Answer from the drawing. Dimensions are ordinates in mm from the lowest x, y and z of the part. Round coordinates to 2 decimals unless told otherwise and drop trailing zeros. Order: outer loops, then holes, each group sorted by start corner. A loop starts at its lowest first (then second) coordinate and runs counter-clockwise, first axis right, second up. Notation, with made-up numbers: (4.25, 43.25) -> (13.25, 43.25) arc R18 ccw to (13.25, 54.25) -> close; hole circle Ø4 at (57, 80). An arc over 180 degrees is marked (long way). Use a Markdown table: item, result. Add a question column.
1. Section D-D, the plane x = 2 is taken. Give the vertices of the cut face in (y, z) (1 decimal).
2. Given pin 1 (4 mm diameter, centred on x = 3.5, z = 59, fed in from +Y); pin 2 (6 mm diameter, centred on y = 3.5, z = 57, fed in from -X); pin 3 (1.5 mm diameter, centred on y = 4, z = 45, fed in from +X); pin 4 (4.5 mm diameter, centred on x = 7.33, y = 6.35, fed in from +Z), each flat-ended and moving along its own axis, determine where each tip first touches the part or whether it passes through.
3. Section C-C, the plane x = 12.5 is taken. Give the vertices of the cut face in (y, z).
4. Consider L1, parallel to Y at x = 11, z = 83.5 (1 decimal); L2, parallel to Y at x = 5.5, z = 109 (1 decimal); L3, parallel to X at y = 5, z = 77 (1 decimal). Determine where each line is inside the solid, lowest interval first. Write a range as [from, to].
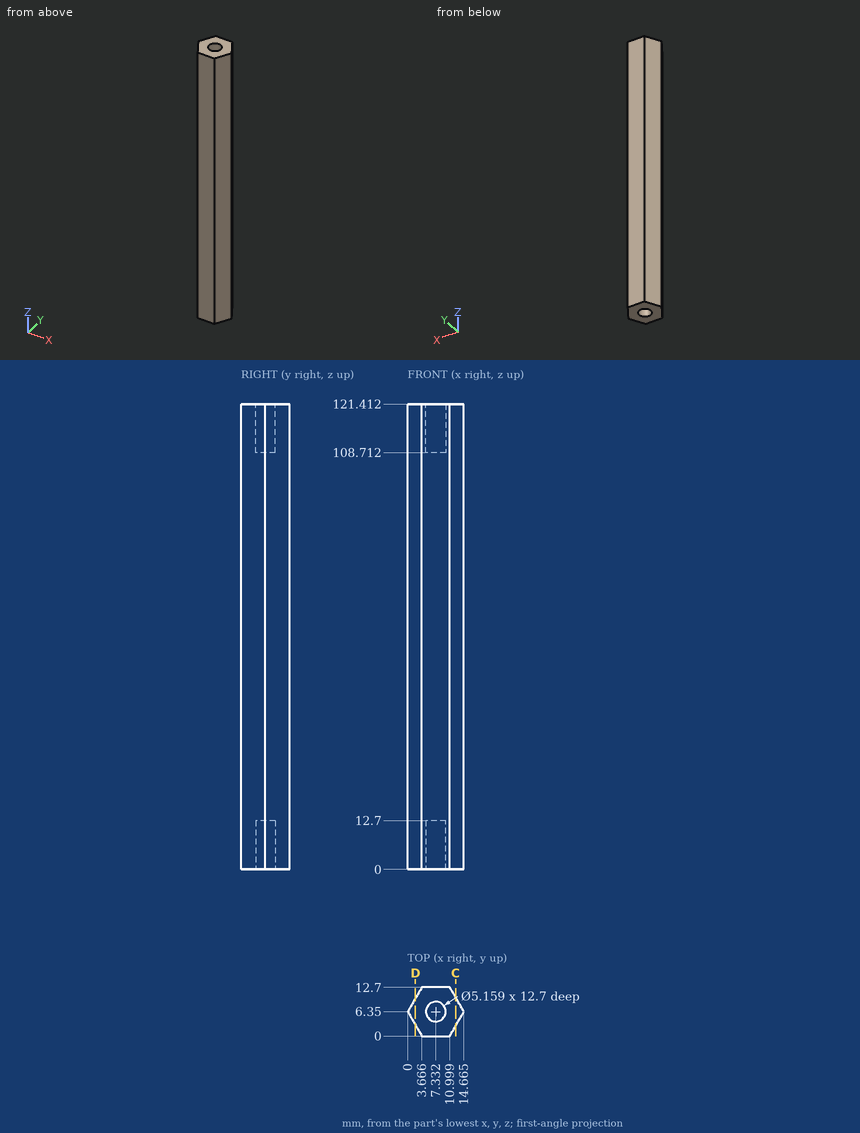
Verdict:
| question | item | result |
|---|---|---|
| 1 | outline | (2.9, 0) -> (9.8, 0) -> (9.8, 121.4) -> (2.9, 121.4) -> close |
| 2 | pin 1 | stops at y = 12.7 |
| 2 | pin 2 | stops at x = 0 |
| 2 | pin 3 | stops at x = 13.74 |
| 2 | pin 4 | stops at z = 108.71 |
| 3 | outline | (2.6, 0) -> (10.1, 0) -> (10.1, 121.41) -> (2.6, 121.41) -> close |
| 4 | L1 | y = [0, 12.7] |
| 4 | L2 | y = [0, 4.5], [8.2, 12.7] |
| 4 | L3 | x = [0.8, 13.9] |
